Source: CAD feature listing. Evaluate the final solid. Frame: model axes, mm. Face numbers are marked on the shaded views. A direction names the side the tool comes from. Give positions to 0.01 mm unless a question says otherwise; leave off trailing zeros. Order: outer loops, then holes, each group sorted by start corner. A loop starts at its lowest first (then second) coordinate and runs counter-clockwise, first axis right, second up. Notation, with made-up numbers: M 15,44.25 L 70,44.25 A19 cw 70,49.25 Z; hole C -9.5,-12 d7. An arc over 180 degrees is marked long. Use CSV: the item, a comma, the result in double quotes. Start each with the question number.
1. Section query C-C, the plane y = -1. Return the cut outline in (x, z).
2. Section query A-A, the plane z = 17.25. Return the cut outline in (x, y), plus the area to 3 significant figures.
3. Reachability of the marked faces 1 and 2 from +Z, -Z, +X, -X, +Y, -Y: full face, straight path, thin tool, end or side. Return the list, or none.
4. Mould query, pull axis X, two halves, no side actions, for the marked faces 3, 4, 5 and 6. Classes: released by +X, released by -X, zero draft, split by the parting line, or undercut.
5. Line query: line 1 along Y through (x, z) = (-6.5, 21.5); line 2 along X through (y, z) = (15.5, 13.75); line 3 along Z through (x, y) = (-22.5, 18). Output: solid intervals per line, ascending. Write a range as [from, to].
6. Pin query (flat end, axial travel): P1, Ø1.5, axis at y = -11, z = 20.5, coming from the +X side; P2, Ø10, axis at x = -57, y = 19, coming from the +Z side. Return the tip coordinate at first contact, or that it passes through.
7. Section query B-B, the plane x = -14.5. Return the cut outline in (y, z).
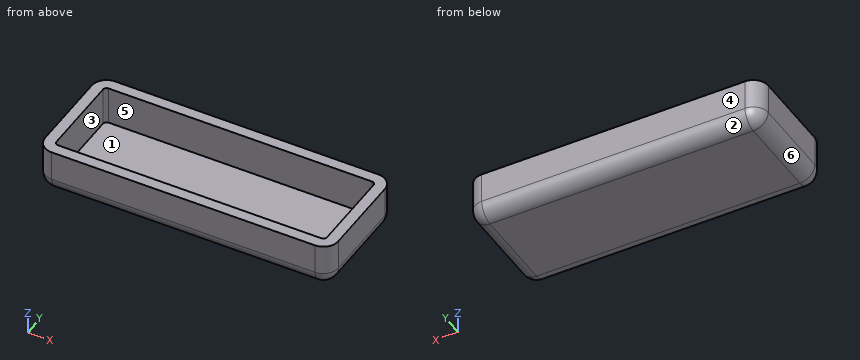
from build123d import *

# Parameters (mm, degrees)
F0_W     = 165.1
F0_H     = 63.5
F1_DEPTH = 25.4
F2_R     = 8.382
F4_DEPTH = 21.59


with BuildPart() as f1:
    # F0 (on Top) → F1 (new body)
    with BuildSketch(Plane.XY):
        with Locations((9.026632, 13.618593)):
            Rectangle(F0_W, F0_H)
    extrude(amount=F1_DEPTH)

    # F2
    f2_edges = [f1.edges().sort_by_distance(p)[0] for p in [
        (91.576632, -18.131407, 12.7),
        (91.576632, 45.368593, 12.7),
        (-73.523368, 45.368593, 12.7),
        (-73.523368, -18.131407, 12.7),
        (9.026632, 45.368593, 0),
        (-73.523368, 13.618593, 0),
        (9.026632, -18.131407, 0),
        (91.576632, 13.618593, 0),
    ]]
    fillet(f2_edges, radius=F2_R)

    # F3 (on face) → F4 (cut)
    with BuildSketch(Plane.XY.offset(25.4)):
        with BuildLine():
            Line((85.226632, -9.749407), (85.226632, 36.986593))
            ThreePointArc((85.226632, 36.986593), (84.631473, 38.423434), (83.194632, 39.018593))
            Line((83.194632, 39.018593), (-65.141368, 39.018593))
            ThreePointArc((-65.141368, 39.018593), (-66.578209, 38.423434), (-67.173368, 36.986593))
            Line((-67.173368, 36.986593), (-67.173368, -9.749407))
            ThreePointArc((-67.173368, -9.749407), (-66.578209, -11.186248), (-65.141368, -11.781407))
            Line((-65.141368, -11.781407), (83.194632, -11.781407))
            ThreePointArc((83.194632, -11.781407), (84.631473, -11.186248), (85.226632, -9.749407))
        make_face()
    extrude(amount=-F4_DEPTH, mode=Mode.SUBTRACT)


solid = f1.part
Result set:
1,outline,"M -73.52,8.38 A8.38 ccw -65.14,0 L 83.19,0 A8.38 ccw 91.58,8.38 L 91.58,25.4 L 85.23,25.4 L 85.23,3.81 L -67.17,3.81 L -67.17,25.4 L -73.52,25.4 Z"
2,outline,"M -73.52,-9.75 A8.38 ccw -65.14,-18.13 L 83.19,-18.13 A8.38 ccw 91.58,-9.75 L 91.58,36.99 A8.38 ccw 83.19,45.37 L -65.14,45.37 A8.38 ccw -73.52,36.99 Z; hole M -67.17,-9.75 A2.03 ccw -65.14,-11.78 L 83.19,-11.78 A2.03 ccw 85.23,-9.75 L 85.23,36.99 A2.03 ccw 83.19,39.02 L -65.14,39.02 A2.03 ccw -67.17,36.99 Z"
2,area,"2,690 mm2"
3,face 1,"+Z"
3,face 2,"-Z, +X, -X, +Y"
4,face 3,"undercut"
4,face 4,"zero draft"
4,face 5,"undercut"
4,face 6,"released by -X"
5,line 1,"[-18.13, -11.78], [39.02, 45.37]"
5,line 2,"[-73.52, -67.17], [85.23, 91.58]"
5,line 3,"[0, 3.81]"
6,P1,"x = 91.56"
6,P2,"z = 3.81"
7,outline,"M -18.13,8.38 A8.38 ccw -9.75,0 L 36.99,0 A8.38 ccw 45.37,8.38 L 45.37,25.4 L 39.02,25.4 L 39.02,3.81 L -11.78,3.81 L -11.78,25.4 L -18.13,25.4 Z"
